Source: CAD feature listing. Evaluate the final solid. Frame: model axes, mm. A direction names the side the tool comes from. Give positions to 0.01 mm unless a question says otherwise; leave off trailing zeros. Loops run counter-clockwise (first coordinate to the right, second up) from the corner with the lowest first, then second, coordinate; pieces in that order, holes last.
```python
from build123d import *

# Parameters (mm, degrees)
F0_R     = 65.3266665863
F0_R_2   = 14.2206371293
F1_DEPTH = 25.4
F3_DEPTH = 78.232
F4_R     = 4.6434374505
F5_DEPTH = 4.064
F6_R     = 3.1082181898
F7_DEPTH = 28.956


with BuildPart() as f1:
    # F0 (on Front) → F1 (new body)
    with BuildSketch(Plane.XZ):
        Circle(F0_R)
        with Locations((-29.2034186423, 33.5097238421)):
            Circle(F0_R_2, mode=Mode.SUBTRACT)
        with Locations((20.3968770802, 36.4621244371)):
            Circle(F0_R_2, mode=Mode.SUBTRACT)
    extrude(amount=F1_DEPTH)

    # F2 (on face) → F3 (join)
    with BuildSketch(Plane.XZ.offset(25.4)):
        Polygon((13.5469222441, -13.4018808603), (0, 9.6108745784), (-18.5700003058, -13.4018808603), align=None)
    extrude(amount=F3_DEPTH)

    # F4 (on face) → F5 (join)
    with BuildSketch(Plane(origin=(4.2016325623, 0, 2.4733756795), x_dir=(0, 1, 0), z_dir=(0.8617703987, 0, 0.5072985117))):
        with Locations((-86.6145864129, -5.7229381055)):
            Circle(F4_R)
    extrude(amount=F5_DEPTH)

    # F6 (on face) → F7 (cut)
    with BuildSketch(Plane(origin=(0, 0, -13.4018808603), x_dir=(1, 0, 0), z_dir=(0, 0, -1))):
        with Locations((-10.1804379374, 95.2019169927)):
            Circle(F6_R)
        with Locations((6.03983727, 95.2019169927)):
            Circle(F6_R)
    extrude(amount=-F7_DEPTH, mode=Mode.SUBTRACT)


solid = f1.part
```
(1) Section B-B, the plane z = -9.5. Return the cut outline in (x, y).
A:
outline: (-64.63, -25.4) - (-15.42, -25.4) - (-15.42, -103.63) - (11.25, -103.63) - (11.25, -25.4) - (64.63, -25.4) - (64.63, 0) - (-64.63, 0) - close; hole circle Ø6.22 at (-10.18, -95.2); hole circle Ø6.22 at (6.04, -95.2)
(2) First-contact query: pin 1 (4 mm diameter, centred on x = 29, y = -27, fed in from +Z); pin 2 (8 mm diameter, centred on x = -10.18, y = -95.2, fed in from -Z); pin 3 (1.5 mm diameter, centred on x = 44, z = -33, fed in from -Y). Flat tips, straight axial feed; report the tip coordinate or a pass-through.
A:
pin 1: stops at z = 59.12
pin 2: stops at z = -13.4
pin 3: stops at y = -25.4
(3) Section D-D, the plane y = -9. Return the cut outline in (x, z), then the cut area to 3 significant figures.
A:
outline: circle Ø130.65 at (0, 0); hole circle Ø28.44 at (-29.2, 33.51); hole circle Ø28.44 at (20.4, 36.46)
area: 12,100 mm2
(4) Ray query, line 1 along X through (y, z) = (-22, 46.5); line 2 along Y through (x, z) = (-41, 3.5); line 3 along Z through (x, y) = (-41, -16). Return the intervals inside material, ascending.
A:
line 1: x = -45.88 to -34.99, -23.42 to 10.32, 30.47 to 45.88
line 2: y = -25.4 to 0
line 3: z = -50.86 to 25.57, 41.45 to 50.86
(5) Section C-C, the plane y = -69. Return the cut outline in (x, z).
A:
outline: (-18.57, -13.4) - (13.55, -13.4) - (0, 9.61) - close
(6) Mould query, pull axis Z, two halves, no side actions, for faces 1 (the flat face through (-3, -103.632, -7)), 2 (the cylindrical face through (10.26, -90.3, -3.88)), 3 (the cylindrical face through (-51.84, -12.52, -39.75)), 4 (the cylindrical face through (28.042, -12.522, 48.453)). Classes: pulls with the +Z half, pulls with the -Z half, needs draft (parallel to the pull), parting line crosses it, or undercut.
A:
face 1: needs draft
face 2: undercut
face 3: parting line crosses it
face 4: undercut
(7) Section A-A, the plane x = -31. Return the cut outline in (y, z), then the cut area to 3 significant figures.
A:
outline: (-25.4, -57.5) - (0, -57.5) - (0, 19.4) - (-25.4, 19.4) - close; (-25.4, 47.62) - (0, 47.62) - (0, 57.5) - (-25.4, 57.5) - close
area: 2,200 mm2
(8) Reachability of faces 5 (the flat face through (-9.155, -63.968, -1.734)), 6 (the flat face through (-3, -64, -13.402)), 7 (the flat face through (10.574, -86.68, -0.341)), 8 (the cylindrical face through (-7.31, -94.01, -7.96)) from +Z, -Z, +X, -X, +Y, -Y: full face, straight path, thin tool, end or side. Return the list, or none.
A:
face 5: +Z, -X, -Y
face 6: -Z, +X, -X, -Y
face 7: +Z, +X, -Y
face 8: +Z, -Z
